Study the drawing (mm; zero at the part's minimum x, y, z) and answer. A direction names the side the tool comes from. Coordinates: 2 decimals unless noted, no trailing zeros. Write each loop counter-clockwise with the first axis right and the second up, starting at its lowest first coordinate (ties: lowest second). Pieces come first, ordered by that corner, then holes. Notation, with made-up numbers: M 79.25,4 L 103.25,4 A21 ccw 103.25,32 Z; hole C -4.5,8.5 d3. An arc over 180 degrees is marked long. Answer as CSV lines item,"result". Start each with the question number.
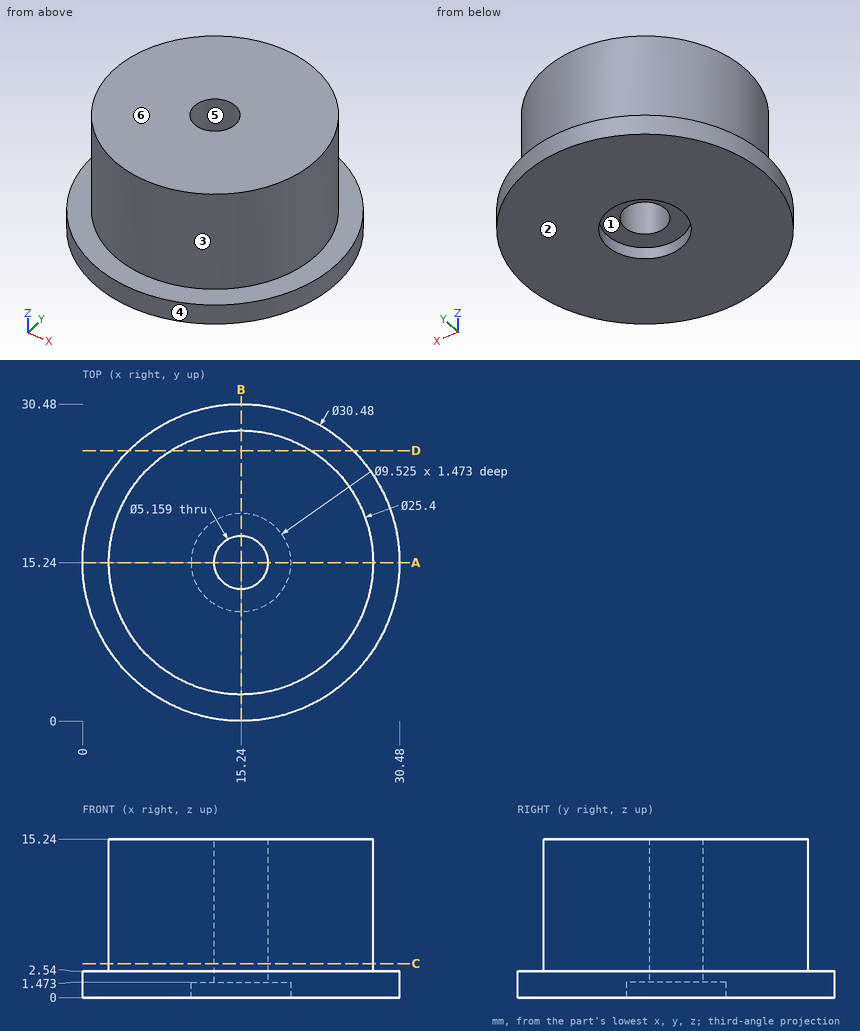
1) Which of the six approach directions +Z, -Z, +X, -X, +Y, -Y give full straight-line access (tool end or side, diameter ignored) to the marked faces 1, 2 and 3?
2) The part is cut by section D-D (y = 26). Determine the outline of the cut face in (x, z), then the cut area to 3 significant figures.
3) For a pull along Y with two mould halves and no side action, classify the marked faces 4, 5 and 6 as +Y half, -Y half, draft (parallel to the pull), parting line (faces both ways), or undercut.
4) Find the intervals of material crossed by line 1 (Y direction, x = 15.24, z = 7.5); line 2 (Y direction, x = 15.24, z = 1.05); line 3 (Z direction, x = 28.5, y = 11), in increasing order. Write a range as from..to.
5) The part is cut by section A-A (y = 15.24). Determine the outline of the cut face in (x, z).
6) Each of these flat-tipped pins is pushed along its axis until it touches: P1, Ø6, axis at x = 15.24, y = 15.24, coming from the -Z side; P2, Ø1, axis at x = 13, z = 5, coming from the -Y side; P3, Ø5, axis at x = 20.5, z = 13, coming from the +Y side. Where does it stop, or does it pass through?
7) The part is cut by section C-C (z = 3.25). Determine the outline of the cut face in (x, y), then the cut area to 3 significant figures.
Completed:
1,face 1,"-Z"
1,face 2,"-Z, +X, -X, +Y, -Y"
1,face 3,"+Z"
2,outline,"M 4.45,0 L 26.03,0 L 26.03,2.54 L 21.99,2.54 L 21.99,15.24 L 8.49,15.24 L 8.49,2.54 L 4.45,2.54 Z"
2,area,"226 mm²"
3,face 4,"parting line"
3,face 5,"undercut"
3,face 6,"draft"
4,line 1,"2.54..12.66, 17.82..27.94"
4,line 2,"0..10.48, 20..30.48"
4,line 3,"0..2.54"
5,outline,"M 0,0 L 10.48,0 L 10.48,1.47 L 12.66,1.47 L 12.66,15.24 L 2.54,15.24 L 2.54,2.54 L 0,2.54 Z; M 17.82,1.47 L 20,1.47 L 20,0 L 30.48,0 L 30.48,2.54 L 27.94,2.54 L 27.94,15.24 L 17.82,15.24 Z"
6,P1,"z = 1.47"
6,P2,"y = 2.66"
6,P3,"y = 27.64"
7,outline,"C 15.24,15.24 d25.4; hole C 15.24,15.24 d5.16"
7,area,"486 mm²"
